Check sheet for the modelled part. Datum: model origin and axes. Units: mm. Face numbers are marked on the shaded views. Coordinates: 2 decimals unless noted, no trailing zeros. Order: outer loops, then holes, each group sorted by start corner. A loop starts at its lowest first (then second) coordinate and runs counter-clockwise, first axis right, second up.
1. Gauge pin test, flat ends, axial feed: pin 1 Ø2 at (y, z) = (36, 7.5) entering from +X; pin 2 Ø1.5 at (x, z) = (91, 7.5) entering from -Y; pin 3 Ø2 at (x, y) = (60.5, 41.5) entering from +Z. Record the tip position at first contact, or that the pin passes through.
2. Draft check along X on the marked faces 1 and 2. Enter one of: released by +X, released by -X, zero draft, split by the parting line, or undercut.
3. Cross-section at B-B (z = 3.25). Count the separate pieces of the cut face and the enclosed holes in it, then the cut area to 3 significant figures.
4. Thickness scan on line 1 (X direction, y = 27, z = 0.75); line 2 (X direction, y = 46, z = 3.75); line 3 (Y direction, x = 67.5, z = 3.75). Record the ranges inside material, lowest first.
5. Cross-section at A-A (x = 157). Enter the section's corners in (y, z), then the cut area to 3 significant figures.
Autodesk Inventor part; units mm, degrees
ref_plane "YZ Plane" through (0, 0, 0) normal (1, 0, 0) x (0, 1, 0)
ref_plane "XZ Plane" through (0, 0, 0) normal (0, 1, 0) x (-1, 0, 0)
ref_plane "XY Plane" through (0, 0, 0) normal (0, 0, 1) x (1, 0, 0)
sketch "Sketch1" plane through (0, 0, 0) normal (0, 0, 1) x (1, 0, 0)
  line L0 (187.5582, 20.5) -> (187.5582, 63.5)
  circle A0 centre (99.5007, 58.7375) radius 2.0955
  line L1 (174.2232, 59.6265) -> (182.4782, 59.6265)
  arc A1 (182.4782, 56.4515) -> (182.4782, 59.6265) centre (182.4782, 58.039) ccw
  line L2 (182.4782, 56.4515) -> (174.2232, 56.4515)
  arc A2 (174.2232, 59.6265) -> (174.2232, 56.4515) centre (174.2232, 58.039) ccw
  line L3 (143.2352, 59.6265) -> (151.4902, 59.6265)
  arc A3 (151.4902, 56.4515) -> (151.4902, 59.6265) centre (151.4902, 58.039) ccw
  line L4 (151.4902, 56.4515) -> (143.2352, 56.4515)
  arc A4 (143.2352, 59.6265) -> (143.2352, 56.4515) centre (143.2352, 58.039) ccw
  circle A5 centre (130.6347, 53.34) radius 4.4
  line L5 (143.2352, 28.6385) -> (151.4902, 28.6385)
  arc A6 (151.4902, 25.4635) -> (151.4902, 28.6385) centre (151.4902, 27.051) ccw
  line L6 (151.4902, 25.4635) -> (143.2352, 25.4635)
  arc A7 (143.2352, 28.6385) -> (143.2352, 25.4635) centre (143.2352, 27.051) ccw
  line L7 (174.2232, 28.6385) -> (182.4782, 28.6385)
  arc A8 (182.4782, 25.4635) -> (182.4782, 28.6385) centre (182.4782, 27.051) ccw
  line L8 (182.4782, 25.4635) -> (174.2232, 25.4635)
  arc A9 (174.2232, 28.6385) -> (174.2232, 25.4635) centre (174.2232, 27.051) ccw
  line L9 (187.5582, 63.5) -> (187.5582, 20.5)
  line L10 (89.6967, 42.545) -> (89.6967, 25.4635)
  circle A10 centre (48.7588, 53.34) radius 4.4
  circle A11 centre (79.8923, 58.737) radius 2.0955
  line L11 (35.9728, 63.5) -> (187.5582, 63.5)
  line L12 (187.5582, 63.5) -> (187.5582, 20.5)
  line L13 (35.9728, 63.5) -> (187.5582, 63.5)
  line L14 (187.5582, 63.5) -> (187.5582, 20.5)
  line L15 (187.5582, 63.5) -> (35.9728, 63.5)
  line L16 (187.5582, 20.5) -> (187.5582, 63.5)
  line L17 (35.9728, 63.5) -> (187.5582, 63.5)
  line L18 (187.5582, 63.5) -> (187.5582, 20.5)
  line L19 (187.5582, 20.5) -> (187.5582, 14.5)
  line L20 (35.9728, 14.5) -> (35.9728, 63.5)
  line L21 (38.7587, 53.34) -> (48.7587, 53.34)
  line L22 (84.6967, 42.545) -> (89.6967, 42.545)
  circle A12 centre (111.7312, 15.24) radius 3.175
  circle A13 centre (97.3962, 12.795) radius 2.2225
  circle A14 centre (81.9972, 12.795) radius 2.2225
  circle A15 centre (67.6622, 15.24) radius 3.175
  circle A16 centre (89.6967, 42.545) radius 4.4
  line L23 (67.6622, 15.24) -> (67.2997, 15.6892)
  line L24 (77.8053, 9.5347) -> (89.6967, 9.5347) construction
  line L25 (111.7312, 15.24) -> (118.0474, 15.24) construction
  line L26 (35.9728, 14.5) -> (35.9728, 9.5)
  line L27 (35.9728, 9.5) -> (187.5582, 9.5)
  line L28 (187.5582, 9.5) -> (187.5582, 14.5)
  circle A17 centre (67.6622, 15.24) radius 3.175
  circle A18 centre (81.9972, 12.795) radius 2.2225
  circle A19 centre (97.3962, 12.795) radius 2.2225
  circle A20 centre (111.7312, 15.24) radius 3.175
  line L29 (165.9682, 54.632) -> (159.6182, 54.632)
  arc A21 (159.6182, 54.632) -> (159.6182, 30.331) centre (159.6182, 42.4815) ccw
  line L30 (159.6182, 30.331) -> (165.9682, 30.331)
  arc A22 (165.9682, 30.331) -> (165.9682, 54.632) centre (165.9682, 42.4815) ccw
  line L31 (80.9972, 12.795) -> (81.9972, 12.795)
  line L32 (98.3962, 12.795) -> (97.3962, 12.795)
  line L33 (76.0442, 58.7375) -> (78.0442, 58.7375)
  line L34 (103.3492, 58.7375) -> (101.3492, 58.7375)
  line L35 (89.6967, 42.545) -> (89.6967, 65.1685)
  line L36 (101.3492, 58.7375) -> (89.6967, 58.7375)
  line L37 (89.6967, 58.7375) -> (79.8923, 58.7375)
  line L38 (165.9682, 42.4815) -> (165.9682, 63.5)
  line L39 (165.9682, 63.5) -> (187.5582, 63.5)
  point P0 (0, 0)
  point P1 (85.6114, 40.9109)
  point P2 (85.5414, 41.0981)
  point P3 (85.3648, 41.7735)
  point P4 (85.4268, 41.4827)
  point P5 (85.6337, 40.856)
  point P6 (85.6114, 44.1791)
  dimension "d4" = 8.8
  dimension "d55" = 10.16
  dimension "d56" = 10.16
  dimension "d57" = 4.7625
  dimension "d58" = 4.763
  dimension "d59" = 20.955
  dimension "d62" = 3.8735
  dimension "d63" = 27.813
  dimension "d66" = 3.8735
  dimension "d67" = 27.813
  dimension "d69" = 10
  dimension "d70" = 5
  dimension "d76" = 8.8
  dimension "d100" = 4.191
  dimension "d101" = 8.8
  dimension "d102" = 1
  dimension "d103" = 1
  dimension "d104" = 2
  dimension "d105" = 2
  dimension "d114" = 9.804
  dimension "d115" = 9.8044
  dimension "d120" = 9.8044
ref_plane "Work Plane6" through (0, 0, 6.35) normal (0, 0, 1) x (1, 0, 0)
extrude "Extrusion18" add sketch "Sketch1" along normal blind 6.35 contours A22 L30 A21 L29 | A16 L10 L35 | L35 L22 A16 | L19 L28 L27 L26 L20 L11 L0 | L22 L10 A16
ref_plane "Work Plane11" through (0, 0, 6.35) normal (0, 0, 1) x (1, 0, 0)
sketch "Sketch9" plane through (0, 0, 6.35) normal (0, 0, 1) x (1, 0, 0)
  circle A0 centre (48.7588, 53.34) radius 4
  line L0 (187.5582, 63.5) -> (25.9728, 63.5)
  arc A1 (44.1657, 63.5) -> (53.3519, 63.5) centre (48.7588, 53.34) ccw
  arc A2 (41.477, 63.5) -> (56.0406, 63.5) centre (48.7588, 53.34) ccw
  point P0 (0, 0)
  dimension "d32" = 22.3
  dimension "d33" = 25
extrude "Extrusion10" add sketch "Sketch9" along normal blind 2 contours A2 L0 A1
ref_plane "Work Plane10" through (0, 0, 6.35) normal (0, 0, 1) x (1, 0, 0)
ref_plane "Work Plane9" through (0, 0, 6.35) normal (0, 0, 1) x (1, 0, 0)
sketch "Sketch11" plane through (0, 0, 6.35) normal (0, 0, 1) x (1, 0, 0)
  circle A0 centre (89.6967, 42.545) radius 4
  circle A1 centre (89.6967, 42.545) radius 11.15
  circle A2 centre (89.6967, 42.545) radius 12.5
  point P0 (0, 0)
  dimension "d40" = 22.3
  dimension "d41" = 25
extrude "Extrusion12" add sketch "Sketch11" along normal blind 2 contours A2
ref_plane "Work Plane7" through (0, 0, 6.35) normal (0, 0, 1) x (1, 0, 0)
ref_plane "Work Plane8" through (0, 0, 6.35) normal (0, 0, 1) x (1, 0, 0)
ref_plane "Work Plane12" through (89.6967, 42.545, 6.35) normal (0, 0, 1) x (1, 0, 0)
sketch "Sketch15" plane through (89.6967, 42.545, 6.35) normal (0, 0, 1) x (1, 0, 0)
  circle A0 centre (0, 0) radius 11.15
  circle A1 centre (0, 0) radius 4
  point P0 (-89.6967, -42.545)
sketch "Sketch17" plane through (0, 0, 6.35) normal (0, 0, 1) x (1, 0, 0)
  arc A0 (44.1657, 63.5) -> (53.3519, 63.5) centre (48.7588, 53.34) ccw
  line L0 (53.3519, 63.5) -> (44.1657, 63.5)
  circle A1 centre (48.7588, 53.34) radius 4.4
  point P0 (0, 0)
extrude "Extrusion22" cut sketch "Sketch17" against normal blind 5
sketch "Sketch10" plane through (0, 0, 6.35) normal (0, 0, 1) x (1, 0, 0)
  line L0 (52.9748, 63.5) -> (56.0406, 63.5)
  circle A0 centre (130.6347, 53.34) radius 4
  arc A1 (126.0415, 63.5) -> (135.2278, 63.5) centre (130.6347, 53.34) ccw
  arc A2 (123.3529, 63.5) -> (137.9164, 63.5) centre (130.6347, 53.34) ccw
  line L1 (187.5582, 63.5) -> (56.0406, 63.5)
  line L2 (123.3529, 63.5) -> (126.0415, 63.5)
  line L3 (135.2278, 63.5) -> (137.9164, 63.5)
  arc A3 (126.0415, 63.5) -> (135.2278, 63.5) centre (130.6347, 53.34) ccw
  arc A4 (123.3529, 63.5) -> (137.9164, 63.5) centre (130.6347, 53.34) ccw
  line L4 (123.3529, 63.5) -> (137.9164, 63.5)
  point P0 (0, 0)
  dimension "d82" = 11.15
extrude "Extrusion26" cut sketch "Sketch10" against normal blind 5 contours L1 A1
sketch "Sketch21" plane through (0, 0, 6.35) normal (0, 0, 1) x (1, 0, 0)
  arc A0 (126.0415, 63.5) -> (135.2278, 63.5) centre (130.6347, 53.34) ccw
  line L0 (126.0415, 63.5) -> (56.0406, 63.5)
  line L1 (187.5582, 63.5) -> (135.2278, 63.5)
  arc A1 (123.3529, 63.5) -> (137.9164, 63.5) centre (130.6347, 53.34) ccw
  line L2 (123.3529, 63.5) -> (126.0415, 63.5)
  line L3 (135.2278, 63.5) -> (137.9164, 63.5)
  point P0 (0, 0)
  dimension "d97" = 25
extrude "Extrusion27" add sketch "Sketch21" along normal blind 2
sketch "Sketch22" plane through (0, 0, 6.35) normal (0, 0, 1) x (1, 0, 0)
  line L0 (35.9728, 63.5) -> (35.9728, 9.5)
  line L1 (35.9728, 9.5) -> (187.5582, 9.5)
  circle A0 centre (39.9728, 13.5) radius 2.2225
  point P0 (0, 0)
  dimension "d106" = 4
  dimension "d107" = 4
extrude "Extrusion28" cut sketch "Sketch22" against normal through all
sketch "Sketch23" plane through (0, 0, 6.35) normal (0, 0, 1) x (1, 0, 0)
  circle A0 centre (39.9728, 13.5) radius 2.2225
  line L0 (35.9728, 9.5) -> (187.5582, 9.5)
  circle A1 centre (138.9208, 13.5) radius 2.2225
  point P0 (0, 0)
  dimension "d110" = 4
  dimension "d111" = 98.948
extrude "Extrusion29" cut sketch "Sketch23" against normal through all contours A1
extrude "Extrusion30" cut sketch "Sketch15" against normal blind 5
sketch "Sketch24" plane through (89.6967, 42.545, 6.35) normal (0, 0, 1) x (1, 0, 0)
  circle A0 centre (0, 0) radius 4
  point P0 (-89.6967, -42.545)
extrude "Extrusion31" cut sketch "Sketch24" against normal through all
sketch "Sketch25" plane through (0, 0, 6.35) normal (0, 0, 1) x (1, 0, 0)
  line L0 (165.9682, 54.632) -> (159.6182, 54.632)
  arc A0 (159.6182, 54.632) -> (159.6182, 30.331) centre (159.6182, 42.4815) ccw
  line L1 (159.6182, 30.331) -> (165.9682, 30.331)
  arc A1 (165.9682, 30.331) -> (165.9682, 54.632) centre (165.9682, 42.4815) ccw
  line L2 (165.9682, 42.4815) -> (165.9682, 63.5)
  line L3 (165.9682, 63.5) -> (187.5582, 63.5)
  point P0 (0, 0)
extrude "Extrusion32" cut sketch "Sketch25" against normal through all
sketch "Sketch26" plane through (0, 0, 6.35) normal (0, 0, 1) x (1, 0, 0)
  line L0 (35.9728, 9.5) -> (187.5582, 9.5)
  circle A0 centre (89.6967, 18.415) radius 5.055
  point P0 (0, 0)
  dimension "d123" = 10.11
  dimension "d124" = 8.915
extrude "Extrusion33" cut sketch "Sketch26" against normal blind 10
sketch "Sketch27" plane through (35.9728, 9.5, 0) normal (-1, 0, 0) x (0, 0, 1)
  line L0 (0, 54) -> (0, 0)
  line L1 (0, 0) -> (6.35, 0)
  line L2 (6.35, 54) -> (6.35, 0)
  line L3 (0, 54) -> (6.35, 54)
  point P0 (0, -9.5)
extrude "Extrusion34" add sketch "Sketch27" along normal blind 8
sketch "Sketch28" plane through (0, 0, 0) normal (0, 0, -1) x (-1, 0, 0)
  line L0 (-187.5582, 63.5) -> (-27.9728, 63.5)
  line L1 (-27.9728, 63.5) -> (-27.9728, 9.5)
  line L2 (-32.0133, 63.5) -> (-32.0133, 34.361)
  line L3 (-32.0133, 56.642) -> (-32.0133, 44.3153) construction
  line L4 (-33.1383, 56.642) -> (-33.1383, 44.3153)
  line L5 (-30.8883, 44.3153) -> (-30.8883, 56.642)
  arc A0 (-30.8883, 56.642) -> (-33.1383, 56.642) centre (-32.0133, 56.642) ccw
  arc A1 (-33.1383, 44.3153) -> (-30.8883, 44.3153) centre (-32.0133, 44.3153) ccw
  point P0 (0, 0)
  point P1 (-32.0133, 50.4786)
  dimension "d129" = 2.25
  dimension "d132" = 6.858
  dimension "d133" = 4.0405
extrude "Extrusion35" cut sketch "Sketch28" against normal blind 8
properties part number "double-left2.0"
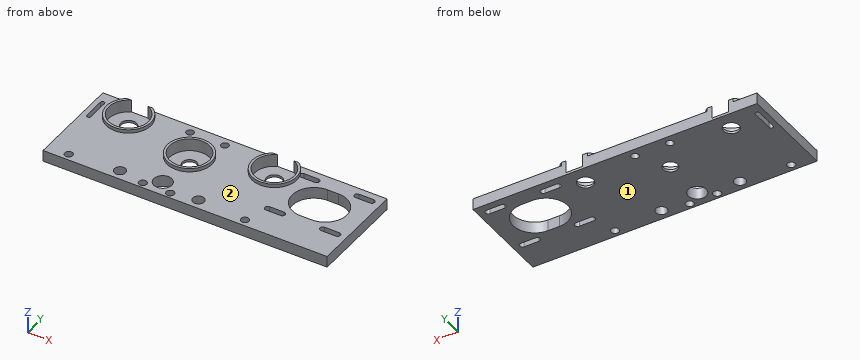
Data:
1. pin 1: stops at x = 100.9
1. pin 2: stops at y = 30.06
1. pin 3: stops at z = 6.35
2. face 1: zero draft
2. face 2: undercut
3. separate pieces: 1
3. enclosed holes: 16
3. area: 6,440 mm2
4. line 1: x = 27.97 to 141.65, 153.08 to 172.64, 184.06 to 187.56
4. line 2: x = 27.97 to 30.89, 33.14 to 40.37, 57.15 to 79.1, 100.3 to 122.24, 139.03 to 147.99, 177.6 to 187.56
4. line 3: y = 9.5 to 12.07, 18.41 to 63.5
5. outline: (9.5, 0) - (30.62, 0) - (30.62, 6.35) - (9.5, 6.35) - close; (54.35, 0) - (63.5, 0) - (63.5, 6.35) - (54.35, 6.35) - close
5. area: 192 mm2
